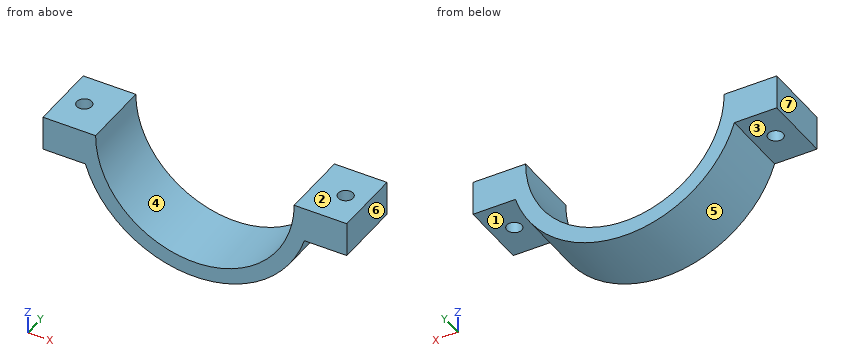
from build123d import *

# Parameters (mm, degrees)
BOSS_EXTRUDE1_DEPTH = 15
SKETCH2_R           = 3.25
CUT_EXTRUDE1_DEPTH  = 77.348743441


with BuildPart() as part:
    # Sketch1 → Boss-Extrude1 (new, symmetric)
    with BuildSketch(Plane(origin=(0, 0, 0), x_dir=(1, 0, 0), z_dir=(0, 1, 0))):
        with BuildLine():
            Line((-66.175, 0), (-66.175, 15))
            Line((-66.175, 15), (-47.696960071, 15))
            ThreePointArc((-47.696960071, 15), (0, 50), (47.696960071, 15))
            Line((47.696960071, 15), (66.175, 15))
            Line((66.175, 15), (66.175, 0))
            Line((66.175, 0), (43.25, 0))
            ThreePointArc((43.25, 0), (0, 43.25), (-43.25, 0))
            Line((-43.25, 0), (-66.175, 0))
        make_face()
    extrude(amount=BOSS_EXTRUDE1_DEPTH, both=True)

    # Sketch2 → Cut-Extrude1 (cut, through all)
    with BuildSketch(Plane(origin=(0, 0, -15), x_dir=(-1, 0, 0), z_dir=(0, 0, -1))):
        with Locations((56.935980035, 0)):
            Circle(SKETCH2_R)
        with Locations((-56.935980035, 0)):
            Circle(SKETCH2_R)
    extrude(amount=-CUT_EXTRUDE1_DEPTH, mode=Mode.SUBTRACT)


solid = part.part
Geometry: final body of the model. Coordinates: model frame, mm. Face numbers are marked on the shaded views. A direction names the side the tool comes from. Round coordinates to 2 decimals unless told otherwise and drop trailing zeros. Loops run counter-clockwise (first coordinate to the right, second up) from the corner with the lowest first, then second, coordinate; pieces in that order, holes last. Notation, with made-up numbers: (-11, 7.5) - (-1, 7.5) arc R8 ccw to (-1, 11.5) - close; hole circle Ø7 at (35.25, 3). An arc over 180 degrees is marked (long way). Write each question's results on one line, items separated by ' | '. Start each with the question number.
1) First-contact query: P1, Ø1, axis at y = 6.5, z = -41, coming from the -X side; P2, Ø8, axis at y = 4.5, z = -33.5, coming from the +X side; P3, Ø10, axis at y = 6, z = -25, coming from the +X side. Flat tips, straight axial feed; report the tip coordinate or a pass-through.
2) Cut plane D-D on z = -17.5. Return loops of the section in (x, y), then the cut area to 3 significant figures.
3) Line query: probe 1 along X at (y, z) = (12, -37.5); probe 2 along X at (y, z) = (11, -23); probe 3 along Z at (x, y) = (52.5, -12). Output: solid intervals per line, ascending. Write a range as [from, to].
4) Mould query, pull axis X, two halves, no side actions, for the marked faces 4, 5, 6 and 7. Classes: released by +X, released by -X, zero draft, split by the parting line, or undercut.
5) Cut plane A-A on z = -6. Return loops of the section in (x, y) (3 decimals), then the cut area to 3 significant figures.
6) Cut plane B-B on y = 0. Return loops of the section in (x, z) (3 decimals), then the cut area to 3 significant figures.
7) Cut plane C-C on x = -56.5. Return loops of the section in (y, z), then the cut area to 3 significant figures.
8) Access query for the marked faces 1, 2 and 3. Directions: +Z, -Z, +X, -X, +Y, -Y. A direction counts if a zero-diameter tool reaches every point of the face in a straight line with its end or side. Return the directions, or none.
Verdict:
1) P1: stops at x = -29.32 | P2: stops at x = 40.37 | P3: stops at x = 45.83
2) outline: (-46.84, -15) - (-39.55, -15) - (-39.55, 15) - (-46.84, 15) - close; (39.55, -15) - (46.84, -15) - (46.84, 15) - (39.55, 15) - close | area: 437 mm2
3) probe 1: x = [-33.07, -21.55], [21.55, 33.07] | probe 2: x = [-44.4, -36.63], [36.63, 44.4] | probe 3: z = [-15, 0]
4) face 4: undercut | face 5: split by the parting line | face 6: released by +X | face 7: released by -X
5) outline: (-66.175, -15) - (-42.832, -15) - (-42.832, 15) - (-66.175, 15) - close; (42.832, -15) - (66.175, -15) - (66.175, 15) - (42.832, 15) - close; hole circle Ø6.5 at (-56.936, 0); hole circle Ø6.5 at (56.936, 0) | area: 1,330 mm2
6) outline: (-66.175, -15) - (-60.186, -15) - (-60.186, 0) - (-66.175, 0) - close; (-53.686, -15) - (-47.697, -15) arc R50 ccw to (47.697, -15) - (53.686, -15) - (53.686, 0) - (43.25, 0) arc R43.25 cw to (-43.25, 0) - (-53.686, 0) - close; (60.186, -15) - (66.175, -15) - (66.175, 0) - (60.186, 0) - close | area: 1,300 mm2
7) outline: (-15, -15) - (-3.22, -15) - (-3.22, 0) - (-15, 0) - close; (3.22, -15) - (15, -15) - (15, 0) - (3.22, 0) - close | area: 353 mm2
8) face 1: -Z, +X, +Y, -Y | face 2: +Z, +X, -X, +Y, -Y | face 3: -Z, -X, +Y, -Y
